Autodesk Inventor part; units mm, degrees
ref_plane "YZ Plane" through (0, 0, 0) normal (1, 0, 0) x (0, 1, 0)
ref_plane "XZ Plane" through (0, 0, 0) normal (0, 1, 0) x (-1, 0, 0)
ref_plane "XY Plane" through (0, 0, 0) normal (0, 0, 1) x (1, 0, 0)
sketch "Sketch1" plane through (0, 0, 0) normal (0, 0, 1) x (1, 0, 0)
  line L0 (0, 0) -> (25.4, 0)
  line L1 (25.4, 0) -> (25.4, 25.4)
  line L2 (25.4, 25.4) -> (0, 25.4)
  line L3 (0, 25.4) -> (0, 0)
  line L4 (1.5875, 1.5875) -> (23.8125, 1.5875)
  line L5 (23.8125, 1.5875) -> (23.8125, 23.8125)
  line L6 (23.8125, 23.8125) -> (1.5875, 23.8125)
  line L7 (1.5875, 23.8125) -> (1.5875, 1.5875)
  dimension "d0" = 25.4
  dimension "d1" = 25.4
  dimension "d2" = 1.5875
extrude "Extrusion1" add sketch "Sketch1" along normal blind 400.05
sketch "Sketch3" plane through (0, 25.4, 0) normal (0, 1, 0) x (1, 0, 0)
  line L0 (25.4, 0) -> (0, 0)
  line L1 (0, 0) -> (0, -400.05)
  line L2 (25.4, -400.05) -> (0, -400.05)
  line L3 (25.4, 0) -> (25.4, -400.05)
  point P0 (0, 0)
  point P1 (12.7, -200.025)
  dimension "d15" = 200.025
  dimension "d16" = 400.05
  dimension "d17" = 12.7
hole "Hole2" at (12.7, 25.4, 200.025) direction (0, -1, 0) diameter 6.35 end through all
sketch "Sketch4" plane through (0, 25.4, 0) normal (0, 1, 0) x (1, 0, 0)
  circle A0 centre (12.7, -200.025) radius 3.175
  line L0 (25.4, 0) -> (0, 0)
  line L1 (0, 0) -> (0, -400.05)
  line L2 (25.4, -400.05) -> (0, -400.05)
  line L3 (25.4, 0) -> (25.4, -400.05)
  point P0 (0, 0)
  point P1 (12.7, -387.35)
  dimension "d25" = 12.7
  dimension "d26" = 12.7
  dimension "d27" = 12.7
hole "Hole3" at (12.7, 25.4, 387.35) direction (0, -1, 0) diameter 6.35 end through all
sketch "Sketch5" plane through (0, 25.4, 0) normal (0, 1, 0) x (1, 0, 0)
  line L0 (25.4, 0) -> (0, 0)
  line L1 (25.4, 0) -> (25.4, -400.05)
  point P0 (12.7, -12.7)
  dimension "d35" = 12.7
  dimension "d36" = 12.7
hole "Hole4" at (12.7, 25.4, 12.7) direction (0, -1, 0) diameter 4.8514 end through all
pattern_linear "Rectangular Pattern1" count 3 spacing 19.05 along (0, 0, 1) of "Hole4"
properties part number "CLB_042_FourPartScissorBarBottom" material "Aluminum 6061"
The model under review builds one solid part; all positions refer to its coordinate system, in mm. A direction names the side the tool comes from. Round coordinates to 2 decimals unless told otherwise and drop trailing zeros. Loops run counter-clockwise (first coordinate to the right, second up) from the corner with the lowest first, then second, coordinate; pieces in that order, holes last. Notation, with made-up numbers: M 21,-26.5 L 66,-26.5 A10 cw 66,-19.5 Z; hole C 72,-12.5 d2. An arc over 180 degrees is marked long. Answer as a JSON object with one key per item and string values.
Item 1: We need section C-C, the plane z = 305.5. State the section outline as (x, y) points, and give its area (3 significant figures).
Check sheet entries:
{"outline": "M 0,0 L 25.4,0 L 25.4,25.4 L 0,25.4 Z; hole M 1.59,1.59 L 23.81,1.59 L 23.81,23.81 L 1.59,23.81 Z", "area": "151 mm2"}
Item 2: We need section A-A, the plane y = 7.25. State the section outline as (x, z) points.
Check sheet entries:
{"outline": "M 0,0 L 1.59,0 L 1.59,400.05 L 0,400.05 Z; M 23.81,0 L 25.4,0 L 25.4,400.05 L 23.81,400.05 Z"}
Item 3: For line 1 along Z through (x, y) = (12.7, 0.85) (3 decimals); line 2 along Y through (x, z) = (14.75, 104); line 3 along X through (y, z) = (0.95, 50.8), list the stretches that pass through material, from the lowest coordinate up.
Check sheet entries:
{"line 1": "0 to 10.274, 15.126 to 29.324, 34.176 to 48.374, 53.226 to 196.85, 203.2 to 384.175, 390.525 to 400.05", "line 2": "0 to 1.59, 23.81 to 25.4", "line 3": "0 to 10.27, 15.13 to 25.4"}
Item 4: The part is to be moulded in two halves that separate along Y. For faces 3 (the face through (1.588, 13, 197)), 4 (the face through (25.4, 13, 197)), 5 (the face through (15, 0, 197)), 6 (the face through (15, 23.812, 197)), say which applies: +Y half, -Y half, draft (parallel to the pull), parting line (faces both ways), or undercut.
Check sheet entries:
{"face 3": "undercut", "face 4": "draft", "face 5": "-Y half", "face 6": "undercut"}
Item 5: Tool access review of faces 1 (the face through (13.916, 0.783, 202.958)), 2 (the face through (10, 1.588, 197)): name each direction out of +Z, -Z, +X, -X, +Y, -Y from which nothing blocks a thin tool from reaching the whole face with its end or side.
Check sheet entries:
{"face 1": "+Y, -Y", "face 2": "+Z, -Z"}
